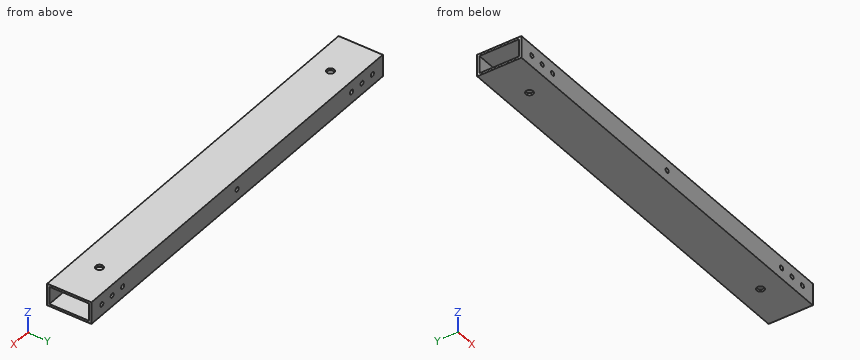
Autodesk Inventor part; units mm, degrees
ref_plane "YZ Plane" through (0, 0, 0) normal (1, 0, 0) x (0, 1, 0)
ref_plane "XZ Plane" through (0, 0, 0) normal (0, 1, 0) x (-1, 0, 0)
ref_plane "XY Plane" through (0, 0, 0) normal (0, 0, 1) x (1, 0, 0)
sketch "スケッチ1" plane through (0, 0, 0) normal (1, 0, 0) x (0, 1, 0)
  line L0 (3.4879, 6.773) -> (-26.5121, 6.773)
  line L1 (-26.5121, 6.773) -> (-26.5121, -8.227)
  line L2 (-26.5121, -8.227) -> (3.4879, -8.227)
  line L3 (3.4879, -8.227) -> (3.4879, 6.773)
  point P0 (0, 0)
  dimension "d0" = 30
  dimension "d1" = 15
extrude "押し出し1" add sketch "スケッチ1" along normal blind 280
sketch "スケッチ2" plane through (0, 3.4879, 6.773) normal (0, 1, 0) x (1, 0, 0)
  circle A0 centre (10, 7.5) radius 1.5
  line L0 (0, 15) -> (0, 0)
  line L1 (0, 15) -> (280, 15)
  circle A1 centre (20, 7.5) radius 1.5
  circle A2 centre (30, 7.5) radius 1.5
  circle A3 centre (270, 7.5) radius 1.5
  line L2 (280, 15) -> (280, 0)
  circle A4 centre (260, 7.5) radius 1.5
  circle A5 centre (250, 7.5) radius 1.5
  point P0 (0, 6.773)
  dimension "d4" = 3
  dimension "d5" = 10
  dimension "d6" = 7.5
  dimension "d7" = 3
  dimension "d8" = 3
  dimension "d9" = 10
  dimension "d10" = 10
  dimension "d11" = 3
  dimension "d12" = 10
  dimension "d13" = 3
  dimension "d14" = 3
  dimension "d15" = 10
  dimension "d16" = 10
hole "穴1" at (270, 3.4879, -0.727) at (260, 3.4879, -0.727) at (250, 3.4879, -0.727) at (10, 3.4879, -0.727) at (20, 3.4879, -0.727) at (30, 3.4879, -0.727) direction (0, -1, 0) diameter 3 depth 30
sketch "スケッチ3" plane through (0, 0, 0) normal (-1, 0, 0) x (0, 0, 1)
  line L0 (-6.727, 1.9879) -> (5.273, 1.9879)
  line L1 (5.273, 1.9879) -> (5.273, -25.0121)
  line L2 (5.273, -25.0121) -> (-6.727, -25.0121)
  line L3 (-6.727, -25.0121) -> (-6.727, 1.9879)
  line L4 (-8.227, 3.4879) -> (6.773, 3.4879)
  line L5 (-8.227, -26.5121) -> (-8.227, 3.4879)
  point P0 (0, 0)
  dimension "d24" = 12
  dimension "d25" = 27
  dimension "d26" = 1.5
  dimension "d27" = 1.5
extrude "押し出し2" cut sketch "スケッチ3" against normal blind 280
sketch "スケッチ4" plane through (0, 3.4879, 6.773) normal (0, 1, 0) x (1, 0, 0)
  circle A0 centre (140, 7.5) radius 1.5
  line L0 (0, 0) -> (280, 0)
  line L1 (0, 15) -> (0, 0)
  point P0 (0, 6.773)
  dimension "d30" = 3
  dimension "d31" = 7.5
  dimension "d32" = 140
hole "穴2" at (140, 3.4879, -0.727) direction (0, -1, 0) diameter 3 depth 30
sketch "スケッチ5" plane through (0, -26.5121, 6.773) normal (0, 0, 1) x (1, 0, 0)
  circle A0 centre (29, 15) radius 2.5
  line L0 (0, 30) -> (0, 0)
  line L1 (0, 30) -> (280, 30)
  point P0 (0, 26.5121)
  dimension "d40" = 5
  dimension "d41" = 29
  dimension "d42" = 15
hole "穴3" at (29, -11.5121, 6.773) direction (0, 0, -1) diameter 5 depth 15
sketch "スケッチ6" plane through (0, -26.5121, 6.773) normal (0, 0, 1) x (1, 0, 0)
  circle A0 centre (251, 15) radius 2.5
  line L0 (280, 30) -> (280, 0)
  line L1 (0, 30) -> (280, 30)
  point P0 (0, 26.5121)
  dimension "d50" = 5
  dimension "d51" = 29
  dimension "d52" = 15
hole "穴4" at (251, -11.5121, 6.773) direction (0, 0, -1) diameter 5 depth 15
equation "\"BendRadius\" = Thickness"
equation "\"BendReliefWidth\" = Thickness"
equation "\"BendReliefDepth\" = 0.5 * Thickness"
equation "\"CornerReliefSize\" = 4 * Thickness"
equation "\"MinimumRemnant\" = 2 * Thickness"
equation "\"TransitionRadius\" = BendRadius"
equation "\"JacobiRadiusSize\" = BendRadius"
equation "\"GapSize\" = Thickness"
properties part number "nhk18" material "アルミニウム 6061"
For this review, take the finished solid that the model builds, in its own axes (mm). Coordinates: 2 decimals unless noted, no trailing zeros. Loops run counter-clockwise (first coordinate to the right, second up) from the corner with the lowest first, then second, coordinate; pieces in that order, holes last. Notation, with made-up numbers: (17, 66.5) - (58, 66.5) arc R20 cw to (58, 99.5) - close; hole circle Ø9 at (-23, 43.5). An arc over 180 degrees is marked (long way). Use one line per item in the form item = value. Start each with the question number.
1) To check wall thickness, follow probe 1 along Z at (x, y) = (70, -19); probe 2 along Z at (x, y) = (270, 2.7); probe 3 along Y at (x, z) = (251, 5.8). State the ranges of each line that lie inside material, in increasing order. Write a range as from..to.
2) Take a section at A-A (y = -19.25). State the section outline as (x, z) points.
3) For pin 1 (2.5 mm diameter, centred on x = 270, z = -0.727, fed in from +Y), flat-tipped, find the tip position at first contact; note if it passes through.
4) Take a section at B-B (x = 57). State the section outline as (y, z) points.
From the geometry:
q1.probe_1 = -8.23..-6.73, 5.27..6.77
q1.probe_2 = -8.23..-2.23, 0.77..6.77
q1.probe_3 = -26.51..-14.01, -9.01..3.49
q2.outline = (0, -8.23) - (280, -8.23) - (280, -6.73) - (0, -6.73) - close; (0, 5.27) - (280, 5.27) - (280, 6.77) - (0, 6.77) - close
q3.pin_1 = through
q4.outline = (-26.51, -8.23) - (3.49, -8.23) - (3.49, 6.77) - (-26.51, 6.77) - close; hole (-25.01, -6.73) - (1.99, -6.73) - (1.99, 5.27) - (-25.01, 5.27) - close
